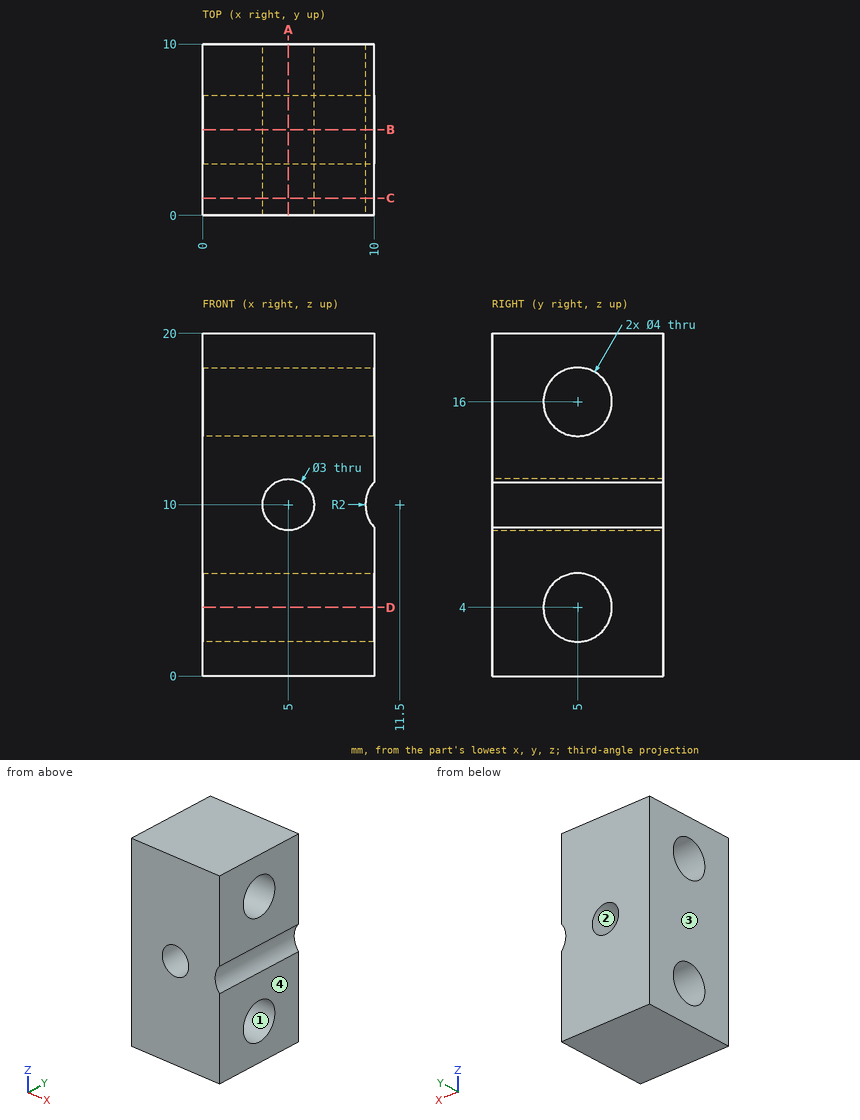
Answer from the drawing. Dimensions are ordinates in mm from the lowest x, y and z of the part. Give positions to 0.01 mm unless a question says otherwise; leave off trailing zeros. Order: outer loops, then holes, each group sorted by start corner. A loop starts at its lowest first (then second) coordinate and runs counter-clockwise, first axis right, second up.
(1) For a pull along X with two mould halves and no side action, classify the marked faces 1, 2, 3 and 4 as released by +X, released by -X, zero draft, split by the parting line, or undercut.
(2) Given pin 1 (4 mm diameter, centred on x = 7.5, z = 9, fed in from -Y), flat-ended and moving along its own axis, determine where the tip first touches the part or whether it passes through.
(3) Find section A-A (x = 5). Give the vertices of the cut face in (y, z), plus the area to 3 significant figures.
(4) Straight lines are drawn through the part: L1, parallel to X at y = 7.75, z = 10; L2, parallel to Y at x = 6.5, z = 4; L3, parallel to Y at x = 6.25, z = 16.75. For each, find the intervals that lie inside material, in ascending order.
(5) Find section B-B (y = 5). Give the vertices of the cut face in (x, z).
(6) Find section D-D (z = 4). Give the vertices of the cut face in (x, y).
(7) Find section C-C (y = 1). Give the vertices of the cut face in (x, z).
Result sheet:
1. face 1: zero draft
1. face 2: undercut
1. face 3: released by -X
1. face 4: released by +X
2. pin 1: stops at y = 0
3. outline: (0, 0) - (10, 0) - (10, 8.5) - (0, 8.5) - close; (0, 11.5) - (10, 11.5) - (10, 20) - (0, 20) - close; hole circle Ø4 at (5, 4); hole circle Ø4 at (5, 16)
3. area: 145 mm2
4. L1: x = 0 to 3.5, 6.5 to 9.5
4. L2: y = 0 to 3, 7 to 10
4. L3: y = 0 to 3.15, 6.85 to 10
5. outline: (0, 0) - (10, 0) - (10, 2) - (0, 2) - close; (0, 6) - (10, 6) - (10, 8.68) arc R2 cw to (10, 11.32) - (10, 14) - (0, 14) - close; (0, 18) - (10, 18) - (10, 20) - (0, 20) - close; hole circle Ø3 at (5, 10)
6. outline: (0, 0) - (10, 0) - (10, 3) - (0, 3) - close; (0, 7) - (10, 7) - (10, 10) - (0, 10) - close
7. outline: (0, 0) - (10, 0) - (10, 8.68) arc R2 cw to (10, 11.32) - (10, 20) - (0, 20) - close; hole circle Ø3 at (5, 10)
